Autodesk Inventor part; units mm, degrees
ref_plane "YZ Plane" through (0, 0, 0) normal (1, 0, 0) x (0, 1, 0)
ref_plane "XZ Plane" through (0, 0, 0) normal (0, 1, 0) x (-1, 0, 0)
ref_plane "XY Plane" through (0, 0, 0) normal (0, 0, 1) x (1, 0, 0)
sketch "Boceto1" plane through (0, 0, 0) normal (1, 0, 0) x (0, 1, 0)
  line L0 (-18.15, 26) -> (18.15, 26)
  line L1 (18.15, 26) -> (18.15, -26)
  line L2 (18.15, -26) -> (-18.15, -26)
  line L3 (-18.15, -26) -> (-18.15, 26)
  line L4 (-18.15, 26) -> (18.15, -26) construction
  line L5 (18.15, 26) -> (-18.15, -26) construction
  point P0 (0, 0)
  dimension "d0" = 36.3
  dimension "d1" = 52
extrude "Extrusión1" add sketch "Boceto1" along normal blind 3
sketch "Boceto2" plane through (3, 0, 0) normal (1, 0, 0) x (0, 0, -1)
  line L0 (-15.7403, 3.1561) -> (-6.6575, 3.1561)
  line L1 (-6.6575, 3.1561) -> (-6.6575, 13.5365)
  line L2 (-6.6575, 13.5365) -> (-15.7403, 13.5365)
  line L3 (-15.7403, 13.5365) -> (-15.7403, 3.1561)
  line L4 (-15.7403, 3.1561) -> (-6.6575, 13.5365) construction
  line L5 (-6.6575, 3.1561) -> (-15.7403, 13.5365) construction
  point P0 (0, 0)
  point P1 (-11.1989, 8.3463)
extrude "Extrusión2" add sketch "Boceto2" along normal blind 0.1
fillet "Empalme1" radius 3 4 edges at (3.05, 13.5365, 15.7403) (3.05, 13.5365, 6.6575) (3.05, 3.1561, 15.7403) (3.05, 3.1561, 6.6575)
mirror "Simetría1" about plane through (0, 0, 0) normal (0, 0, 1) of "Extrusión2", "Empalme1"
properties part number "pantalla"
Design review of the part built by this model. Coordinates are the model's own, in mm. Coordinates: 2 decimals unless noted, no trailing zeros. Write each loop counter-clockwise with the first axis right and the second up, starting at its lowest first coordinate (ties: lowest second). Pieces come first, ordered by that corner, then holes.
1) Add section A-A (y = 9). Write out the cut boundary in (x, z).
2) Add section C-C (y = 4). Write out the cut boundary in (x, z), plus the area to 3 significant figures.
3) To check wall thickness, follow L1, parallel to X at y = 7.5, z = -0.5. State the ranges of the line that lie inside material, in increasing order.
4) Add section B-B (z = 10.5). Write out the cut boundary in (x, y), plus the area to 3 significant figures.
5) Insertion check: pin 1 (1.5 mm diameter, centred on y = 11, z = -3.5, fed in from +X). The pin has a flat end and moves straight along its axis. Give the tip position at first contact, or say it passes through.
6) Add section D-D (z = -20.5). Write out the cut boundary in (x, y).
Check result:
1. outline: (0, -26) - (3, -26) - (3, -15.74) - (3.1, -15.74) - (3.1, -6.66) - (3, -6.66) - (3, 6.66) - (3.1, 6.66) - (3.1, 15.74) - (3, 15.74) - (3, 26) - (0, 26) - close
2. outline: (0, -26) - (3, -26) - (3, -14.83) - (3.1, -14.83) - (3.1, -7.57) - (3, -7.57) - (3, 7.57) - (3.1, 7.57) - (3.1, 14.83) - (3, 14.83) - (3, 26) - (0, 26) - close
2. area: 157 mm2
3. L1: x = 0 to 3
4. outline: (0, -18.15) - (3, -18.15) - (3, 3.16) - (3.1, 3.16) - (3.1, 13.54) - (3, 13.54) - (3, 18.15) - (0, 18.15) - close
4. area: 110 mm2
5. pin 1: stops at x = 3
6. outline: (0, -18.15) - (3, -18.15) - (3, 18.15) - (0, 18.15) - close
